Source: three-view drawing plus pictorial views. Frame: mm from the lowest corner of the part. A direction names the side the tool comes from. Coordinates: 2 decimals unless noted, no trailing zeros. Loops run counter-clockwise (first coordinate to the right, second up) from the corner with the lowest first, then second, coordinate; pieces in that order, holes last.
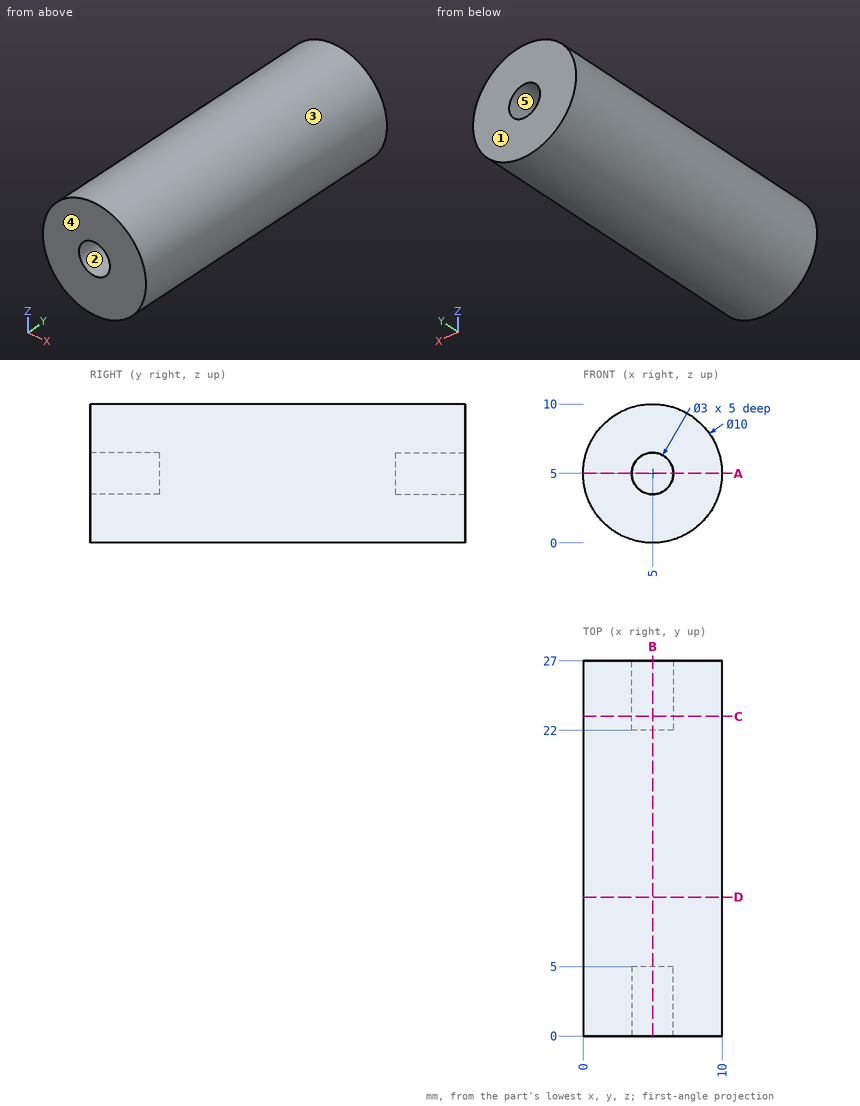
Q1. Draft query along Z for the marked faces 1, 2 and 3. Return one class per face: released by +Z, released by -Z, zero draft, split by the parting line, or undercut.
Q2. Section query A-A on z = 5. Return the cut outline in (x, y), then the cut area to 3 significant figures.
Q3. Section query D-D on y = 10. Return the cut outline in (x, z).
Q4. Reachability of the marked faces 4 and 5 from +Z, -Z, +X, -X, +Y, -Y: full face, straight path, thin tool, end or side. Return the list, or none.
Q5. Section query C-C on y = 23. Return the cut outline in (x, z).
Q6. First-contact query: pin 1 Ø5 at (x, z) = (5, 5) entering from +Y; pin 2 Ø1 at (x, y) = (2.5, 3) entering from +Z; pin 3 Ø2.5 at (x, z) = (5, 5) entering from +Y; pin 4 Ø2 at (x, y) = (2, 15.5) entering from -Z. Flat tips, straight axial feed; report the tip coordinate or a pass-through.
Q7. Section query B-B on x = 5. Return the cut outline in (y, z).
Q8. Material intervals for line 1 along Z through (x, y) = (5, 1.35); line 2 along Z through (x, y) = (6.25, 1.75), sorted ascending.
Resolved:
1. face 1: zero draft
1. face 2: undercut
1. face 3: split by the parting line
2. outline: (0, 0) - (3.5, 0) - (3.5, 5) - (6.5, 5) - (6.5, 0) - (10, 0) - (10, 27) - (6.5, 27) - (6.5, 22) - (3.5, 22) - (3.5, 27) - (0, 27) - close
2. area: 240 mm2
3. outline: circle Ø10 at (5, 5)
4. face 4: +Z, -Z, +X, -X, -Y
4. face 5: +Y
5. outline: circle Ø10 at (5, 5); hole circle Ø3 at (5, 5)
6. pin 1: stops at y = 27
6. pin 2: stops at z = 9.58
6. pin 3: stops at y = 22
6. pin 4: stops at z = 0.42
7. outline: (0, 0) - (27, 0) - (27, 3.5) - (22, 3.5) - (22, 6.5) - (27, 6.5) - (27, 10) - (0, 10) - (0, 6.5) - (5, 6.5) - (5, 3.5) - (0, 3.5) - close
8. line 1: z = 0 to 3.5, 6.5 to 10
8. line 2: z = 0.16 to 4.17, 5.83 to 9.84
